Autodesk Inventor part; units mm, degrees
ref_plane "YZ Plane" through (0, 0, 0) normal (1, 0, 0) x (0, 1, 0)
ref_plane "XZ Plane" through (0, 0, 0) normal (0, 1, 0) x (-1, 0, 0)
ref_plane "XY Plane" through (0, 0, 0) normal (0, 0, 1) x (1, 0, 0)
sketch "Sketch1" plane through (0, 0, 0) normal (0, 0, 1) x (1, 0, 0)
  line L0 (-15, -15) -> (-15, 15)
  line L1 (-15, 15) -> (15, 15)
  line L2 (15, 15) -> (15, -15)
  line L3 (15, -15) -> (-15, 15) construction
  line L4 (-15, -15) -> (15, 15) construction
  line L5 (0, 0) -> (8.0802, 0) construction
  line L6 (0, 0) -> (0, 7.2946) construction
  line L7 (-5.05, -20.05) -> (5.05, -20.05)
  line L8 (5.05, -20.05) -> (5.05, -9.95)
  line L9 (5.05, -9.95) -> (-5.05, -9.95)
  line L10 (-5.05, -9.95) -> (-5.05, -20.05)
  line L11 (-5.05, -20.05) -> (5.05, -9.95) construction
  line L12 (5.05, -20.05) -> (-5.05, -9.95) construction
  line L13 (15, -15) -> (5.05, -15)
  line L14 (-5.05, -15) -> (-15, -15)
  point P0 (-12, -12.5)
  point P1 (12, -12.5)
  point P2 (-12, 12.5)
  point P3 (12, 12.5)
  point P4 (0, -15)
  dimension "d0" = 30
  dimension "d1" = 30
  dimension "d4" = 24
  dimension "d7" = 25
  dimension "d10" = 10.1
  dimension "d11" = 10.1
extrude "Extrusion1" add sketch "Sketch1" along normal blind 15 contours L0 L1 L2 L13 L8 L9 L10 L14
hole "Hole1" at (12, 12.5, 0) at (-12, 12.5, 0) at (-12, -12.5, 0) at (12, -12.5, 0) direction (0, 0, 1) diameter 2.9 end through all
sketch "Sketch2" plane through (0, 0, 0) normal (0, 0, -1) x (-1, 0, 0)
  point P0 (0, 0)
  point P1 (0, 0)
hole "Hole2" at (0, 0, 0) direction (0, 0, 1) diameter 5.3 end through all
sketch "Sketch3" plane through (0, 0, 15) normal (0, 0, 1) x (1, 0, 0)
  line L0 (15, 15) -> (-15, 15)
  line L1 (-15, 15) -> (-9, 15)
  line L2 (-9, 15) -> (-9, 10)
  line L3 (-9, 10) -> (-15, 10)
  line L4 (-15, 10) -> (-15, 15)
  line L5 (15, -15) -> (15, 15)
  line L6 (15, 15) -> (9, 15)
  line L7 (9, 15) -> (9, 10)
  line L8 (9, 10) -> (15, 10)
  line L9 (15, 10) -> (15, 15)
  line L10 (-15, -15) -> (-5.05, -15)
  line L11 (-15, -15) -> (-9, -15)
  line L12 (-9, -15) -> (-9, -10)
  line L13 (-9, -10) -> (-15, -10)
  line L14 (-15, -10) -> (-15, -15)
  line L15 (15, -15) -> (9, -15)
  line L16 (9, -15) -> (9, -10)
  line L17 (9, -10) -> (15, -10)
  line L18 (15, -10) -> (15, -15)
  circle A0 centre (0, 0) radius 2.65
  circle A1 centre (-12, -12.5) radius 1.45
  circle A2 centre (12, 12.5) radius 1.45
  circle A3 centre (-12, 12.5) radius 1.45
  circle A4 centre (12, -12.5) radius 1.45
  line L19 (15, 15) -> (-15, 15)
  line L20 (-15, 15) -> (-15, -15)
  line L21 (-15, -15) -> (-5.05, -15)
  line L22 (-5.05, -15) -> (-5.05, -9.95)
  line L23 (-5.05, -9.95) -> (5.05, -9.95)
  line L24 (5.05, -9.95) -> (5.05, -15)
  line L25 (5.05, -15) -> (15, -15)
  line L26 (15, -15) -> (15, 15)
  dimension "d28" = 6
  dimension "d29" = 5
  dimension "d30" = 6
  dimension "d31" = 5
  dimension "d32" = 6
  dimension "d33" = 5
extrude "Extrusion2" cut sketch "Sketch3" against normal blind 2 contours L7 L8 L5 L17 L16 L25 L24 L23 L22 L10 L12 L13 L20 L3 L2 L0
sketch "Sketch4" plane through (0, 0, 13) normal (0, 0, 1) x (1, 0, 0)
  line L0 (2.3671, 4.1) -> (4.7343, 0)
  line L1 (4.7343, 0) -> (2.3671, -4.1)
  line L2 (2.3671, -4.1) -> (-2.3671, -4.1)
  line L3 (-2.3671, -4.1) -> (-4.7343, 0)
  line L4 (-4.7343, 0) -> (-2.3671, 4.1)
  line L5 (-2.3671, 4.1) -> (2.3671, 4.1)
  point P0 (0, 0)
  point P1 (0, 0)
  dimension "d36" = 8.2
extrude "Extrusion3" cut sketch "Sketch4" against normal blind 10
properties part number "front_door-webcam(FIT0701)-mount"
Part model, mm, in its own coordinate system. A direction names the side the tool comes from. Coordinates: 2 decimals unless noted, no trailing zeros. Write each loop counter-clockwise with the first axis right and the second up, starting at its lowest first coordinate (ties: lowest second). Pieces come first, ordered by that corner, then holes. Notation, with made-up numbers: (65.25, -32) - (76.25, -32) arc R26 ccw to (76.25, 4) - close; hole circle Ø2 at (55, -1.75). An arc over 180 degrees is marked (long way). Put each result on its own line as item: value.
1. Band-saw the part on D-D (z = 1.75). Write the cut outline in (x, y), then the cut area to 3 significant figures.
Final values:
outline: (-15, -15) - (-5.05, -15) - (-5.05, -9.95) - (5.05, -9.95) - (5.05, -15) - (15, -15) - (15, 15) - (-15, 15) - close; hole circle Ø2.9 at (-12, -12.5); hole circle Ø2.9 at (-12, 12.5); hole circle Ø5.3 at (0, 0); hole circle Ø2.9 at (12, -12.5); hole circle Ø2.9 at (12, 12.5)
area: 801 mm²
2. Band-saw the part on A-A (z = 7). Write the cut outline in (x, y), then the cut area to 3 significant figures.
Final values:
outline: (-15, -15) - (-5.05, -15) - (-5.05, -9.95) - (5.05, -9.95) - (5.05, -15) - (15, -15) - (15, 15) - (-15, 15) - close; hole circle Ø2.9 at (-12, -12.5); hole circle Ø2.9 at (-12, 12.5); hole (-4.73, 0) - (-2.37, -4.1) - (2.37, -4.1) - (4.73, 0) - (2.37, 4.1) - (-2.37, 4.1) - close; hole circle Ø2.9 at (12, -12.5); hole circle Ø2.9 at (12, 12.5)
area: 764 mm²
3. Flat gauge pins, fed straight in: pin 1 Ø2.5 at (x, y) = (12, 12.5) entering from -Z; pin 2 Ø6.5 at (x, y) = (2, 1) entering from +Z; pin 3 Ø4 at (x, z) = (-1, 10.5) entering from -Y. Where does each tip first touch, or does it go through?
Final values:
pin 1: passes through
pin 2: stops at z = 13
pin 3: stops at y = -9.95
4. Band-saw the part on B-B (x = 12). Write the cut outline in (y, z), then the cut area to 3 significant figures.
Final values:
outline: (-15, 0) - (-13.95, 0) - (-13.95, 15) - (-15, 15) - close; (-11.05, 0) - (11.05, 0) - (11.05, 15) - (10, 15) - (10, 13) - (-10, 13) - (-10, 15) - (-11.05, 15) - close; (13.95, 0) - (15, 0) - (15, 15) - (13.95, 15) - close
area: 323 mm²
5. 3-axis set-ups, long thin cutter, end or side, ignore diameter. For faces 5 (the flat face through (3.57, -2.02, 8.07)), 6 (the flat face through (-9, 13, 14)), 7 (the flat face through (-15, 0, 7)), 8 (the flat face through (12, 10, 14)): which of +Z, -Z, +X, -X, +Y, -Y reach the whole face in a straight line?
Final values:
face 5: +Z
face 6: +Z, +Y, -Y
face 7: +Z, -Z, -X, +Y, -Y
face 8: +Z, +X, -X
6. Band-saw the part on C-C (x = 0). Write the cut outline in (y, z), then the cut area to 3 significant figures.
Final values:
outline: (-9.95, 0) - (-2.65, 0) - (-2.65, 3) - (-4.1, 3) - (-4.1, 13) - (-9.95, 13) - close; (2.65, 0) - (15, 0) - (15, 13) - (4.1, 13) - (4.1, 3) - (2.65, 3) - close
area: 226 mm²
7. Probe line 1 along Y through (x, z) = (12, 9.25); line 2 along X through (y, z) = (-12.5, 5.5); line 3 along X through (y, z) = (12.5, 11.5). List the from-to ranges inside material, lowest first. Write a range as [from, to].
Final values:
line 1: y = [-15, -13.95], [-11.05, 11.05], [13.95, 15]
line 2: x = [-15, -13.45], [-10.55, -5.05], [5.05, 10.55], [13.45, 15]
line 3: x = [-15, -13.45], [-10.55, 10.55], [13.45, 15]
8. Two-plate mould, pull along Y, no slides. Class faces 1 (the flat face through (2, 2, 3)), 2 (the flat face through (-3.57, 2.02, 8.07)), 3 (the flat face through (0, -9.95, 6)), 4 (the flat face through (15, 0, 7)): +Y half, -Y half, draft (parallel to the pull), parting line (faces both ways), or undercut.
Final values:
face 1: undercut
face 2: undercut
face 3: -Y half
face 4: draft
